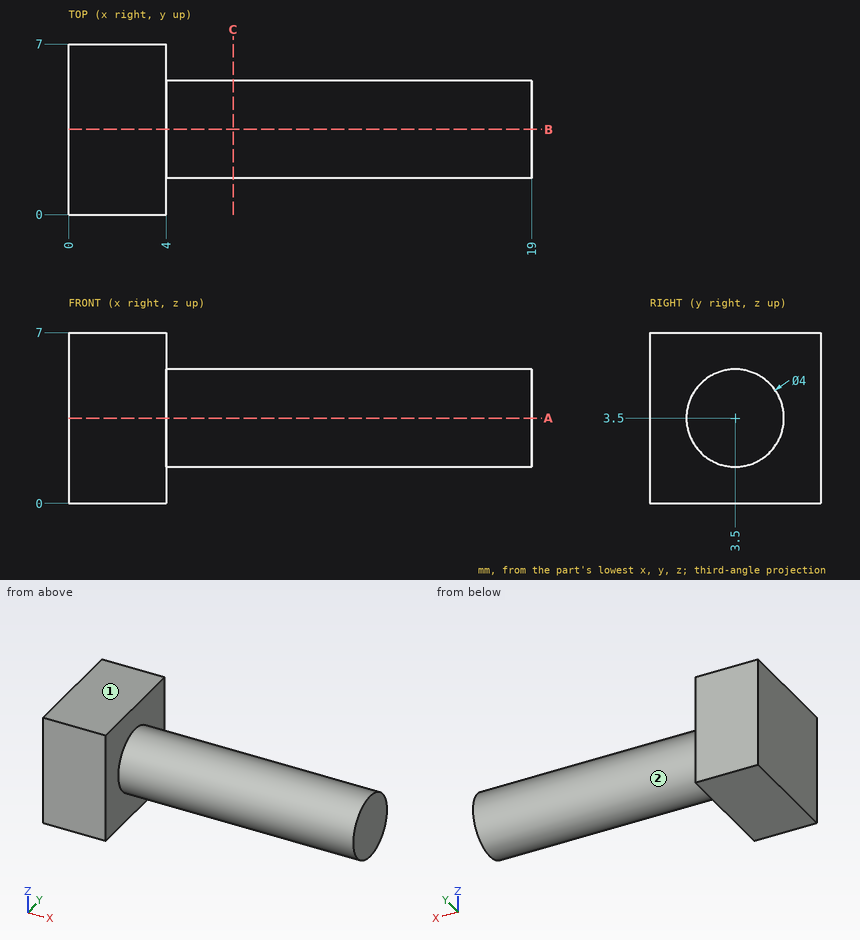
Here's the drawing with two shaded views (mm, measured from the low corner). I have some questions. A direction names the side the tool comes from. Give positions to 0.01 mm unless a question says otherwise; leave off trailing zeros. Loops run counter-clockwise (first coordinate to the right, second up) from the corner with the lowest first, then second, coordinate; pieces in that order, holes last. Notation, with made-up numbers: (5, 2) - (62, 2) arc R15 cw to (62, 20) - close; hole circle Ø9 at (53, -24). An arc over 180 degrees is marked (long way). One line per item, written item: value.
(1) I'm going to push flat-ended pins straight in: pin 1 (1.5 mm diameter, centred on x = 11, z = 2, fed in from +Y); pin 2 (1 mm diameter, centred on y = 6.5, z = 5.5, fed in from +X); pin 3 (4 mm diameter, centred on x = 7, z = 2, fed in from -Y). Where does each tip first touch, or does it pass through?
Verdict:
pin 1: y = 5.35
pin 2: x = 4
pin 3: y = 1.5
(2) I need wall thicknesses on line 1 along X through (y, z) = (5, 5); line 2 along Y through (x, z) = (17, 3.5); line 3 along Y through (x, z) = (14.5, 5.25). Which ranges of each line are inside material? Lowest first, please.
Verdict:
line 1: 0 to 4
line 2: 1.5 to 5.5
line 3: 2.53 to 4.47
(3) If we section it at A-A, the plane z = 3.5: List the corners of the cut face in (x, y) for me, plus the area to 3 significant figures.
Verdict:
outline: (0, 0) - (4, 0) - (4, 1.5) - (19, 1.5) - (19, 5.5) - (4, 5.5) - (4, 7) - (0, 7) - close
area: 88.0 mm^2
(4) On a 3-axis mill with a long thin cutter (end or side, diameter ignored), from which of +Z, -Z, +X, -X, +Y, -Y can I reach the whole of each face in a straight line? I mean the marked faces 1 and 2. Say none if no direction works.
Verdict:
face 1: +Z, +X, -X, +Y, -Y
face 2: +X
(5) If we section it at C-C, the plane x = 6.75: List the corners of the cut face in (y, z) for me, plus the area to 3 significant figures.
Verdict:
outline: circle Ø4 at (3.5, 3.5)
area: 12.6 mm^2
